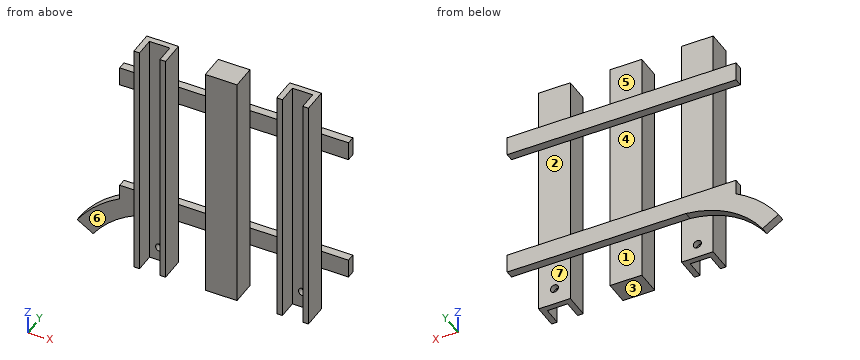
Autodesk Inventor part; units mm, degrees
ref_plane "Work Plane2" through (32.2, 0, -89.46) normal (-1, 0, 0) x (0, 0, 1)
ref_plane "YZ Plane" through (0, 0, 0) normal (1, 0, 0) x (0, 1, 0)
ref_plane "XZ Plane" through (0, 0, 0) normal (0, 1, 0) x (-1, 0, 0)
sketch "Sketch1" plane through (0, 0, 0) normal (0, 1, 0) x (-1, 0, 0)
  line L0 (0, 0) -> (-11.7, 0)
  line L1 (-11.7, 0) -> (-11.7, -89.46)
  line L2 (-11.7, -89.46) -> (0, -89.46)
  line L3 (0, -89.46) -> (0, 0)
  line L4 (-26.35, 0) -> (-38.05, 0)
  line L5 (-38.05, 0) -> (-38.05, -89.46)
  line L6 (-38.05, -89.46) -> (-26.35, -89.46)
  line L7 (-26.35, -89.46) -> (-26.35, 0)
  line L8 (-52.7, 0) -> (-64.4, 0)
  line L9 (-64.4, 0) -> (-64.4, -89.46)
  line L10 (-64.4, -89.46) -> (-52.7, -89.46)
  line L11 (-52.7, -89.46) -> (-52.7, 0)
  dimension "d0" = 11.7
  dimension "d1" = 11.7
  dimension "d2" = 11.7
  dimension "d3" = 14.65
  dimension "d4" = 14.65
  dimension "d5" = 89.46
  dimension "d47" = 64.4
extrude "Extrusion1" add sketch "Sketch1" along normal blind 9
sketch "Sketch2" plane through (0, 9, 0) normal (0, 1, 0) x (1, 0, 0)
  line L0 (38.05, 89.46) -> (26.35, 89.46) construction
  line L1 (32.2, 89.46) -> (32.2, 0) construction
  line L2 (26.35, 0) -> (38.05, 0) construction
  line L3 (11.7, 89.46) -> (0, 89.46) construction
  line L4 (5.85, 89.46) -> (5.85, 0) construction
  line L5 (0, 0) -> (11.7, 0) construction
  circle A0 centre (5.85, 84.16) radius 1.5
  line L6 (52.7, 0) -> (64.4, 0) construction
  line L7 (58.55, 0) -> (58.55, 89.46) construction
  circle A1 centre (58.55, 83.16) radius 1.5
  line L8 (64.4, 89.46) -> (52.7, 89.46) construction
  dimension "d8" = 3
  dimension "d9" = 5.3
  dimension "d50" = 3
  dimension "d51" = 6.3
extrude "Extrusion2" cut sketch "Sketch2" against normal blind 8
sketch "Sketch3" plane through (11.7, 0, -89.46) normal (0, 0, -1) x (-1, 0, 0)
  line L0 (-14.65, 9) -> (-26.35, 9) construction
  line L1 (-20.5, 9) -> (-20.5, 0) construction
  line L2 (-14.65, 0) -> (-26.35, 0) construction
  line L3 (0, 0) -> (11.7, 0)
  line L4 (9.6, 0) -> (9.6, 6.9)
  line L5 (9.6, 6.9) -> (2.1, 6.9)
  line L6 (2.1, 6.9) -> (2.1, 0)
  line L7 (2.1, 0) -> (9.6, 0) construction
  line L8 (0, 0) -> (0, 9) construction
  line L9 (11.7, 0) -> (11.7, 9) construction
  line L10 (-41, 0) -> (-52.7, 0)
  line L11 (-50.6, 0) -> (-50.6, 6.9)
  line L12 (-50.6, 6.9) -> (-43.1, 6.9)
  line L13 (-43.1, 6.9) -> (-43.1, 0)
  dimension "d15" = 7.5
  dimension "d16" = 2.1
  dimension "d17" = 2.1
  dimension "d18" = 6.9
extrude "Extrusion3" cut sketch "Sketch3" against normal through all
sketch "Sketch4" plane through (0, 9, 0) normal (0, 1, 0) x (1, 0, 0)
  line L0 (0, 89.46) -> (0, 0) construction
  line L1 (0, 44.73) -> (64.4, 44.73) construction
  line L2 (64.4, 0) -> (64.4, 89.46) construction
  line L3 (-10, 16.9) -> (74.4, 16.9)
  line L4 (74.4, 16.9) -> (74.4, 23.9)
  line L5 (74.4, 23.9) -> (-10, 23.9)
  line L6 (-10, 23.9) -> (-10, 16.9)
  line L7 (-10, 72.56) -> (74.4, 72.56)
  line L8 (74.4, 72.56) -> (74.4, 65.56)
  line L9 (74.4, 65.56) -> (-10, 65.56)
  line L10 (-10, 65.56) -> (-10, 72.56)
  line L11 (52.7, 0) -> (64.4, 0)
  dimension "d21" = 7
  dimension "d22" = 10
  dimension "d23" = 10
  dimension "d46" = 16.9
extrude "Extrusion4" add sketch "Sketch4" along normal blind 3
ref_plane "Work Plane2" through (32.2, 0, -89.46) normal (-1, 0, 0) x (0, 0, 1)
sketch "Sketch8" plane through (0, 9, 0) normal (0, 1, 0) x (1, 0, 0)
  line L0 (74.4, 72.56) -> (-10, 72.56)
  line L1 (-10, 72.56) -> (-10, 65.56)
  line L2 (-10, 65.56) -> (74.4, 65.56)
  line L3 (74.4, 65.56) -> (74.4, 72.56)
  arc A0 (-19.9091, 89.4398) -> (8.4822, 72.56) centre (12.2544, 111.2215) ccw
  arc A1 (-25.6819, 85.5304) -> (8.4822, 65.56) centre (12.2544, 111.2215) ccw
  line L4 (8.4822, 65.56) -> (8.4822, 72.56)
  line L5 (9.6, 89.46) -> (9.6, 0)
  line L6 (-19.7721, 89.2387) -> (-25.6819, 85.5304)
  point P0 (0, 0)
extrude "Extrusion8" add sketch "Sketch8" along normal up to surface (3 mm away) contours L4 A1 L1 L0 | L0 L1 A1 L6 A0
ref_plane "Work Plane3" through (45.375, 0, 0) normal (1, 0, 0) x (0, 0, -1)
sketch "Sketch5" plane through (0, 8.5, 0) normal (0, -1, 0) x (1, 0, 0)
  line L0 (23, -75) -> (14, -75)
  line L1 (14, -75) -> (14, -22)
  line L2 (14, -22) -> (23, -22)
  line L3 (23, -22) -> (23, -75)
  line L4 (26, -90) -> (26, 0)
  line L5 (11, 0) -> (11, -90)
  line L6 (11, -22) -> (26, -22)
  line L7 (11, -68) -> (26, -68)
  point P0 (0, 0)
  point P1 (18.5, -22)
  dimension "d27" = 3
  dimension "d28" = 3
  dimension "d29" = 9
  dimension "d30" = 7
sketch "Sketch6" plane through (23, 8.5, -75) normal (0, 0, -1) x (-1, 0, 0)
  line L0 (9, 0) -> (9, -2)
  line L1 (0, 0) -> (0, -2)
  line L2 (9, -0.5) -> (0, -0.5)
  line L3 (0, -0.5) -> (0, -1.5)
  line L4 (0, -1.5) -> (9, -1.5)
  line L5 (9, -1.5) -> (9, -0.5)
  line L6 (9, 0) -> (0, 0)
  line L7 (9, -2) -> (0, -2)
  point P0 (23, -8.5)
  dimension "d34" = 0.5
  dimension "d35" = 0.5
  dimension "d36" = 1
sketch "Sketch7" plane through (14, 8, -75) normal (0, 1, 0) x (1, 0, 0)
  line L0 (1.5, 2) -> (7.5, 2)
  line L1 (7.5, 2) -> (7.5, 4.5)
  line L2 (7.5, 4.5) -> (1.5, 4.5)
  line L3 (1.5, 4.5) -> (1.5, 2)
  line L4 (0, 0) -> (0, 7)
  line L5 (9, 0) -> (9, 7)
  line L6 (0, 7) -> (9, 7)
  point P0 (-14, -75)
  dimension "d39" = 6
  dimension "d40" = 2.5
  dimension "d41" = 1.5
  dimension "d42" = 1.5
  dimension "d43" = 2.5
equation "\"d1\" = d0"
equation "\"d2\" = d1"
equation "\"d4\" = d3"
equation "\"d17\" = d16"
equation "\"d23\" = d22"
equation "\"d28\" = d27"
equation "\"d35\" = d34"
equation "\"d42\" = d41"
properties part number "tracks"
Can you work these out from the model? Positions are in its coordinate system, mm. Face numbers are marked on the shaded views. A direction names the side the tool comes from. Give positions to 0.01 mm unless a question says otherwise; leave off trailing zeros. Loops run counter-clockwise (first coordinate to the right, second up) from the corner with the lowest first, then second, coordinate; pieces in that order, holes last. Notation, with made-up numbers: (72, 33.5) -> (96, 33.5) arc R12 ccw to (96, 38.5) -> close; hole circle Ø10 at (57.25, 52.5). An arc over 180 degrees is marked (long way). Return JSON: item names as keys, results as strings.
Q1. I want a section at A-A, the plane y = 3.5. List the corners of the cut face in (x, z) for me, then the cut area to 3 significant figures.
Checks:
{"outline": "(0, -89.46) -> (2.1, -89.46) -> (2.1, 0) -> (0, 0) -> close; (9.6, -89.46) -> (11.7, -89.46) -> (11.7, 0) -> (9.6, 0) -> close; (26.35, -89.46) -> (38.05, -89.46) -> (38.05, 0) -> (26.35, 0) -> close; (52.7, -89.46) -> (54.8, -89.46) -> (54.8, 0) -> (52.7, 0) -> close; (62.3, -89.46) -> (64.4, -89.46) -> (64.4, 0) -> (62.3, 0) -> close", "area": "1,800 mm2"}
Q2. We'd pull the mould along Z, two halves only. Please class the marked faces 1, 2 and 3: released by +Z, released by -Z, zero draft, split by the parting line, or undercut.
Checks:
{"face 1": "zero draft", "face 2": "undercut", "face 3": "released by -Z"}
Q3. For pin 1 Ø5.5 at (x, z) = (-6, -20.5) entering from -Y; pin 2 Ø6 at (y, z) = (2.5, -44) entering from -X; pin 3 Ø3.5 at (x, z) = (59, -51.5) entering from +Y, each with a flat end and sliding along its axis, tell me the tip position at first contact or that it passes through.
Checks:
{"pin 1": "stops at y = 9", "pin 2": "stops at x = 0", "pin 3": "stops at y = 9"}
Q4. I want a section at B-B, the plane z = -9.5. List the corners of the cut face in (x, y) for me.
Checks:
{"outline": "(0, 0) -> (2.1, 0) -> (2.1, 6.9) -> (9.6, 6.9) -> (9.6, 0) -> (11.7, 0) -> (11.7, 9) -> (0, 9) -> close; (26.35, 0) -> (38.05, 0) -> (38.05, 9) -> (26.35, 9) -> close; (52.7, 0) -> (54.8, 0) -> (54.8, 6.9) -> (62.3, 6.9) -> (62.3, 0) -> (64.4, 0) -> (64.4, 9) -> (52.7, 9) -> close"}
Q5. On a 3-axis mill with a long thin cutter (end or side, diameter ignored), from which of +Z, -Z, +X, -X, +Y, -Y can I reach the whole of each face in a straight line? I mean the marked faces 4, 5, 6 and 7. Say none if no direction works.
Checks:
{"face 4": "+X, -X, +Y", "face 5": "+Z, +X, -X, +Y", "face 6": "+Z, -Z, -X, -Y", "face 7": "-Z, +X, +Y"}
Q6. I want a section at D-D, the plane x = 34. List the corners of the cut face in (y, z) for me, then the cut area to 3 significant figures.
Checks:
{"outline": "(0, -89.46) -> (9, -89.46) -> (9, -72.56) -> (12, -72.56) -> (12, -65.56) -> (9, -65.56) -> (9, -23.9) -> (12, -23.9) -> (12, -16.9) -> (9, -16.9) -> (9, 0) -> (0, 0) -> close", "area": "847 mm2"}
Q7. I need wall thicknesses on probe 1 along X at (y, z) = (5, -22); probe 2 along X at (y, z) = (8, -33); probe 3 along Z at (x, y) = (58.55, 7.4). Which ranges of each line are inside material? Lowest first, please.
Checks:
{"probe 1": "x = 0 to 2.1, 9.6 to 11.7, 26.35 to 38.05, 52.7 to 54.8, 62.3 to 64.4", "probe 2": "x = 0 to 11.7, 26.35 to 38.05, 52.7 to 64.4", "probe 3": "z = -89.46 to -84.66, -81.66 to 0"}
Q8. I want a section at C-C, the plane x = 58.55. List the corners of the cut face in (y, z) for me.
Checks:
{"outline": "(6.9, -89.46) -> (9, -89.46) -> (9, -84.66) -> (6.9, -84.66) -> close; (6.9, -81.66) -> (9, -81.66) -> (9, -72.56) -> (12, -72.56) -> (12, -65.56) -> (9, -65.56) -> (9, -23.9) -> (12, -23.9) -> (12, -16.9) -> (9, -16.9) -> (9, 0) -> (6.9, 0) -> close"}
